Geometry: final body of the model. Coordinates: model frame, mm. A direction names the side the tool comes from. Give positions to 0.01 mm unless a question says otherwise; leave off trailing zeros. Loops run counter-clockwise (first coordinate to the right, second up) from the corner with the lowest first, then second, coordinate; pieces in that order, holes last. Notation, with made-up numbers: M 46,74 L 80,74 A36 cw 80,111 Z; hole C -22.5,-1.5 d11. An arc over 180 degrees is marked long. Put each result on its own line as item: value.
Autodesk Inventor part; units mm, degrees
ref_plane "YZ Plane" through (0, 0, 0) normal (1, 0, 0) x (0, 1, 0)
ref_plane "XZ Plane" through (0, 0, 0) normal (0, 1, 0) x (-1, 0, 0)
ref_plane "XY Plane" through (0, 0, 0) normal (0, 0, 1) x (1, 0, 0)
sketch "Sketch1" plane through (0, 0, 0) normal (0, 0, 1) x (1, 0, 0)
  circle A0 centre (13, 8.75) radius 1.5
  circle A1 centre (13, -8.75) radius 1.5
  line L0 (9.525, 11.15) -> (16.475, 11.15)
  line L1 (16.475, 11.15) -> (16.475, -16.3)
  line L2 (9.525, 11.15) -> (9.525, -16.3)
  line L3 (9.525, -16.3) -> (16.475, -16.3)
  point P0 (0, 0)
  dimension "d0" = 27.45
  dimension "d1" = 3.475
  dimension "d2" = 2.4
  dimension "d3" = 3.475
extrude "Extrusion1" add sketch "Sketch1" along normal blind 9.5
sketch "Sketch2" plane through (9.525, -16.3, 0) normal (-1, 0, 0) x (0, 0, 1)
  line L0 (0, 27.45) -> (9.5, 27.45)
  line L1 (9.5, 0) -> (9.5, 27.45)
  arc A0 (3, 27.45) -> (9.5, 4) centre (48.5502, 27.45) ccw
  line L2 (0, 27.45) -> (9.5, 27.45)
  point P0 (0, 16.3)
  dimension "d6" = 3
  dimension "d7" = 4
extrude "Extrusion2" cut sketch "Sketch2" against normal blind 10
sketch "Sketch3" plane through (9.525, -16.3, 0) normal (0, -1, 0) x (1, 0, 0)
  line L0 (0, 0) -> (0, 9.5)
  line L1 (0, 0) -> (6.95, 0)
  line L2 (0, 4.75) -> (6.95, 4.75)
  line L3 (6.95, 4.75) -> (6.95, 0)
  line L4 (6.95, 0) -> (0, 0)
  line L5 (0, 0) -> (0, 4.75)
  circle A0 centre (3.855, 7.075) radius 1.375
  point P0 (-9.525, 0)
  dimension "d14" = 3.855
  dimension "d15" = 2.325
  dimension "d16" = 2.75
extrude "Extrusion3" cut sketch "Sketch3" against normal blind 7.9125 contours A0
extrude "Extrusion4" cut sketch "Sketch3" against normal blind 1.25 contours L0 L2 L3 L1
sketch "Sketch4" plane through (0, 0, 9.5) normal (0, 0, 1) x (1, 0, 0)
  circle A0 centre (13, -8.75) radius 3.25
  circle A1 centre (13, 8.75) radius 3.25
  circle A2 centre (13, -8.75) radius 1.5
  circle A3 centre (13, 8.75) radius 1.5
  point P0 (0, 0)
  dimension "d17" = 6.5
extrude "Extrusion5" cut sketch "Sketch4" against normal blind 4.7875 contours A0
extrude "Extrusion6" cut sketch "Sketch4" against normal up to surface (6.5 mm away) contours A1 | A3
properties part number "ENCODERV2PLATE"
Item 1: Section A-A on z = 1.75. Output: boundary loops of the cut face in (x, y) (3 decimals), then the cut area to 3 significant figures.
Output values:
outline: M 9.525,-15.05 L 16.475,-15.05 L 16.475,11.15 L 9.525,11.15 Z; hole C 13,-8.75 d3; hole C 13,8.75 d3
area: 168 mm²
Item 2: Mould query, pull axis Y, two halves, no side actions, for faces 1 (the flat face through (13, -14, 9.5)), 2 (the cylindrical face through (11.81, 9.66, 1.48)), 3 (the flat face through (12, -16.3, 8)). Classes: pulls with the +Y half, pulls with the -Y half, needs draft (parallel to the pull), parting line crosses it, or undercut.
Output values:
face 1: needs draft
face 2: undercut
face 3: pulls with the -Y half
Item 3: Section C-C on x = 13.38. Output: boundary loops of the cut face in (y, z), then the cut area to 3 significant figures.
Output values:
outline: M -16.3,4.75 L -15.05,4.75 L -15.05,0 L -10.2,0 L -10.2,4.71 L -11.98,4.71 L -11.98,5.7 L -16.3,5.7 Z; M -16.3,8.45 L -11.98,8.45 L -11.98,9.31 A45.55 cw -12.3,9.5 L -16.3,9.5 Z; M -7.3,0 L 7.3,0 L 7.3,3 L 5.52,3 L 5.52,3.35 A45.55 cw -5.52,6.16 L -5.52,4.71 L -7.3,4.71 Z; M 10.2,0 L 11.15,0 L 11.15,3 L 10.2,3 Z
area: 97.9 mm²
Item 4: Line query: probe 1 along Y at (x, z) = (13, 1.7); probe 2 along Y at (x, z) = (13, 3.25); probe 3 along Z at (x, y) = (10.5, 9.25). Output: solid intervals per line, ascending. Write a range as [from, to].
Output values:
probe 1: [-15.05, -10.25], [-7.25, 7.25], [10.25, 11.15]
probe 2: [-15.05, -10.25], [-7.25, 5.5]
probe 3: [0, 3]
Item 5: Set-up query: faces 4 (the flat face through (14, -7, 4.712)), 5 (the cylindrical face through (14.69, -13.93, 7.49)), 6 (the flat face through (13, -15.05, 2)). Return all of +Z, -Z, +X, -X, +Y, -Y with unobstructed straight access to the full face (end or side cutting, diameter ignored); none if empty.
Output values:
face 4: +Z
face 5: -Y
face 6: -Z, +X, -X, -Y
Item 6: Section B-B on y = 8.75. Output: boundary loops of the cut face in (x, z) (3 decimals), then the cut area to 3 significant figures.
Output values:
outline: M 9.525,0 L 11.5,0 L 11.5,3 L 9.75,3 L 9.75,3.063 L 9.525,3.063 Z; M 14.5,0 L 16.475,0 L 16.475,3.063 L 16.25,3.063 L 16.25,3 L 14.5,3 Z
area: 11.9 mm²
Item 7: Pin query (flat end, axial travel): pin 1 Ø2.5 at (x, z) = (13.38, 7.075) entering from -Y; pin 2 Ø3 at (x, y) = (14, -8) entering from +Z; pin 3 Ø2.5 at (x, y) = (13, -8.75) entering from +Z; pin 4 Ø1 at (x, y) = (15, 3.5) entering from +Z. Return the tip coordinate at first contact, or that it passes through.
Output values:
pin 1: y = -5.79
pin 2: z = 4.71
pin 3: through
pin 4: z = 3.74
Item 8: Section D-D on y = -13.25. Output: boundary loops of the cut face in (x, z) (3 decimals).
Output values:
outline: M 9.525,0 L 16.475,0 L 16.475,9.5 L 9.525,9.5 Z; hole C 13.38,7.075 d2.75
